Read the model definition and answer for the solid it produces. Units are mm, in the model's axes. A direction names the side the tool comes from. Give positions to 0.01 mm unless a question says otherwise; leave off trailing zeros. Order: outer loops, then holes, each group sorted by start corner. A loop starts at its lowest first (then second) coordinate and runs counter-clockwise, first axis right, second up. Notation, with made-up numbers: (89.5, 85.25) - (116.5, 85.25) arc R18 ccw to (116.5, 111.25) - close; hole circle Ø9 at (41.25, 89.5). An arc over 180 degrees is marked (long way). Use a Markdown table: item, result. Add a question column.
1. Consider L1, parallel to Y at x = -10, z = -113; L2, parallel to Y at x = -17, z = -16. Determine where each line is inside the solid, lowest interval first.
2. A cutting plane is placed at A-A on y = 7.5. State how many separate pieces and enclosed holes the cut face has, and give its area (3 significant figures).
3. A cutting plane is placed at B-B on z = -79. Determine the outline of the cut face in (x, y), and give its area (3 significant figures).
4. Flat-ended cylindrical pins translate along their axes: P1, Ø2, axis at x = -1.5, z = -239.5, coming from the +Y side; P2, Ø5, axis at x = -2, z = -343, coming from the +Y side; P3, Ø4, axis at x = 2.5, z = -155.5, coming from the -Y side; P4, Ø3, axis at x = 4, y = 4, coming from the +Z side. Find the tip coordinate at first contact, or state that the pin passes through.
5. Which of the six approach directions +Z, -Z, +X, -X, +Y, -Y give full straight-line access (tool end or side, diameter ignored) to faces 1 (the flat face through (0.35, 4.756, -208.097)), 2 (the flat face through (-25, 0.3, -161.4)), 3 (the flat face through (0.35, 5.24, -129.01))?
6. For a pull along Z with two mould halves and no side action, classify faces 4 (the flat face through (0.35, 5.244, -208.282)), 5 (the flat face through (0, 5.25, -345)), 6 (the flat face through (0.35, 7.82, -13.31)) as released by +Z, released by -Z, zero draft, split by the parting line, or undercut.
```python
from build123d import *

# Parameters (mm, degrees)
EXTRUDE_THIN1_DEPTH = 25


with BuildPart() as part:
    # Sketch3 → Extrude-Thin1 (new body, symmetric)
    with BuildSketch(Plane(origin=(0, 0, 0), x_dir=(0, 0, -1), z_dir=(1, 0, 0))):
        Polygon((0, 4.75), (10.083940671, 4.75), (16.606328425, 9.686469499), (29.818985275, -0.313530501), (43.031642125, 9.686469499), (56.244298974, -0.313530501), (69.456955824, 9.686469499), (82.669612674, -0.313530501), (95.882269524, 9.686469499), (109.094926374, -0.313530501), (122.307583223, 9.686469499), (135.520240073, -0.313530501), (148.732896923, 9.686469499), (161.945553773, -0.313530501), (175.158210623, 9.686469499), (188.370867472, -0.313530501), (201.583524322, 9.686469499), (214.796181172, -0.313530501), (228.008838022, 9.686469499), (241.221494872, -0.313530501), (254.434151721, 9.686469499), (267.646808571, -0.313530501), (280.859465421, 9.686469499), (294.072122271, -0.313530501), (307.284779121, 9.686469499), (320.49743597, -0.313530501), (333.71009282, 9.686469499), (340.232480575, 4.75), (350.316421245, 4.75), (350.316421245, 5.25), (340.400361916, 5.25), (333.71009282, 10.313530501), (320.49743597, 0.313530501), (307.284779121, 10.313530501), (294.072122271, 0.313530501), (280.859465421, 10.313530501), (267.646808571, 0.313530501), (254.434151721, 10.313530501), (241.221494872, 0.313530501), (228.008838022, 10.313530501), (214.796181172, 0.313530501), (201.583524322, 10.313530501), (188.370867472, 0.313530501), (175.158210623, 10.313530501), (161.945553773, 0.313530501), (148.732896923, 10.313530501), (135.520240073, 0.313530501), (122.307583223, 10.313530501), (109.094926374, 0.313530501), (95.882269524, 10.313530501), (82.669612674, 0.313530501), (69.456955824, 10.313530501), (56.244298974, 0.313530501), (43.031642125, 10.313530501), (29.818985275, 0.313530501), (16.606328425, 10.313530501), (9.916059329, 5.25), (0, 5.25), align=None)
    extrude(amount=EXTRUDE_THIN1_DEPTH, both=True)


solid = part.part
```
Output values:
| question | item | result |
|---|---|---|
| 1 | L1 | 2.64 to 3.27 |
| 1 | L2 | 9.23 to 9.85 |
| 2 | separate pieces | 26 |
| 2 | enclosed holes | 0 |
| 2 | area | 1,080 mm² |
| 3 | outline | (-25, 2.46) - (25, 2.46) - (25, 3.09) - (-25, 3.09) - close |
| 3 | area | 31.4 mm² |
| 4 | P1 | y = 2.37 |
| 4 | P2 | y = 5.25 |
| 4 | P3 | y = 3.05 |
| 4 | P4 | z = 0 |
| 5 | face 1 | +X, -X, -Y |
| 5 | face 2 | +Z, -Z, -X, +Y, -Y |
| 5 | face 3 | +X, -X, +Y |
| 6 | face 4 | undercut |
| 6 | face 5 | zero draft |
| 6 | face 6 | released by +Z |
